The figure shows three views and two pictorial views of one solid part (mm, origin at its lowest corner). Answer the questions. A direction names the side the tool comes from. Give positions to 0.01 mm unless a question says otherwise; leave off trailing zeros. Order: outer loops, then holes, each group sorted by start corner. A loop starts at its lowest first (then second) coordinate and runs counter-clockwise, first axis right, second up. Notation, with made-up numbers: (64.25, 63) - (115.25, 63) arc R28 ccw to (115.25, 84) - close; hole circle Ø11 at (-30.5, 16). An arc over 180 degrees is marked (long way). Answer as CSV lines item,"result". Start each with the question number.
1. Section A-A on z = 28.5 is taken. Give the vertices of the cut face in (x, y).
2. Section B-B on x = 6.5 is taken. Count the separate pieces of the cut face and the enclosed holes in it, and give its area (4 significant figures).
3. Section D-D on z = 6.9 is taken. Give the vertices of the cut face in (x, y).
4. Flat-ended cylindrical pins translate along their axes: pin 1 (2 mm diameter, centred on x = 6.5, z = 24, fed in from +Y); pin 2 (14.5 mm diameter, centred on y = 12.95, z = 6.9, fed in from +X); pin 3 (14.5 mm diameter, centred on x = 29.5, y = 13, fed in from -Z). Find the tip coordinate at first contact, or state that the pin passes through.
5. Which of the six approach directions +Z, -Z, +X, -X, +Y, -Y give full straight-line access (tool end or side, diameter ignored) to the marked faces 5, 6 and 7?
6. Section C-C on y = 22 is taken. Give the vertices of the cut face in (x, z).
7. Consider line 1 along Z through (x, y) = (6.5, 29); line 2 along X through (y, z) = (2.25, 28.5); line 3 along Y through (x, z) = (6.5, 23.25). Determine where each line is inside the solid, lowest interval first. Write a range as [from, to].
8. Determine the mould class of the marked faces 1, 2, 3 and 4 for opening direction Z: +Z half, -Z half, draft (parallel to the pull), parting line (faces both ways), or undercut.
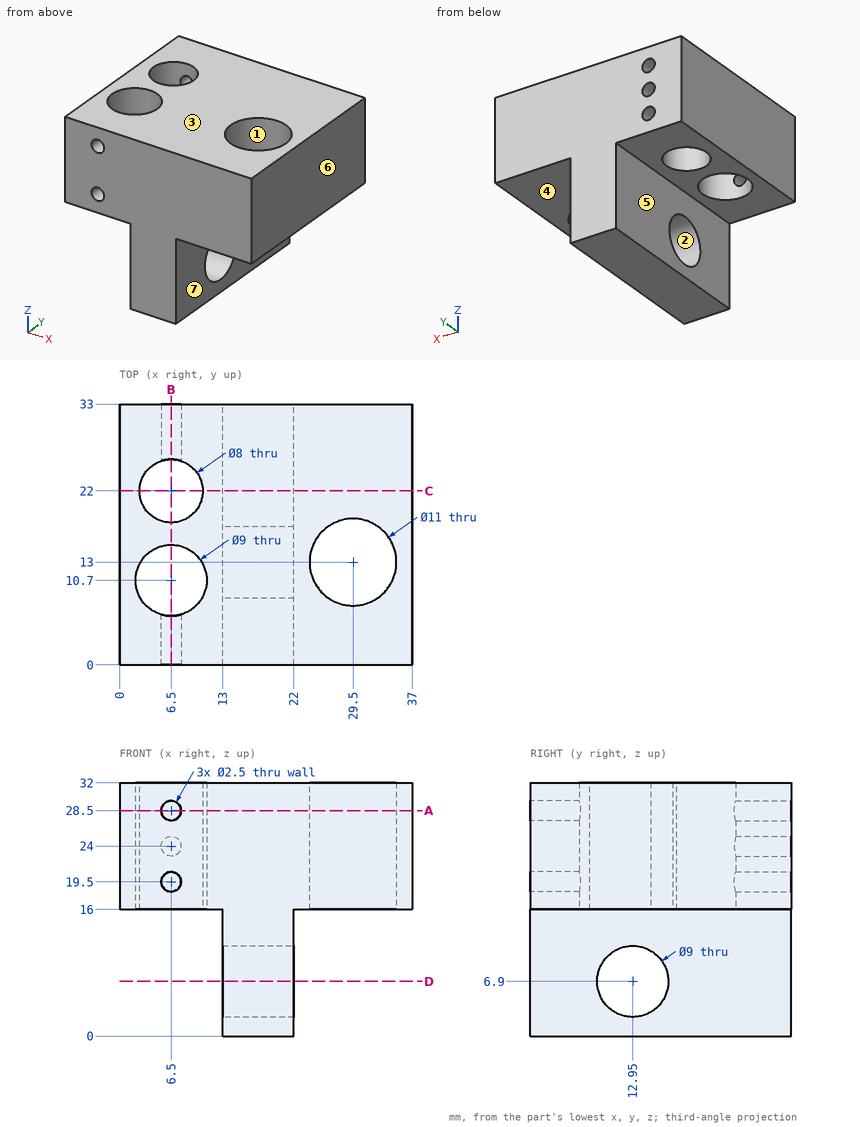
Checks:
1,outline,"(0, 0) - (5.25, 0) - (5.25, 6.38) arc R4.5 cw (long way) to (7.75, 6.38) - (7.75, 0) - (37, 0) - (37, 33) - (7.75, 33) - (7.75, 25.8) arc R4 cw (long way) to (5.25, 25.8) - (5.25, 33) - (0, 33) - close; hole circle Ø11 at (29.5, 13)"
2,separate pieces,"8"
2,enclosed holes,"0"
2,area,"172.5 mm²"
3,outline,"(13, 0) - (22, 0) - (22, 8.45) - (13, 8.45) - close; (13, 17.45) - (22, 17.45) - (22, 33) - (13, 33) - close"
4,pin 1,"stops at y = 18.13"
4,pin 2,"stops at x = 22"
4,pin 3,"stops at z = 16"
5,face 5,"-Z, -X, +Y, -Y"
5,face 6,"+Z, -Z, +X, +Y, -Y"
5,face 7,"-Z, +X, +Y, -Y"
6,outline,"(0, 16) - (2.5, 16) - (2.5, 32) - (0, 32) - close; (10.5, 16) - (13, 16) - (13, 0) - (22, 0) - (22, 16) - (37, 16) - (37, 32) - (10.5, 32) - close"
7,line 1,"z = [16, 18.25], [20.75, 22.75], [25.25, 27.25], [29.75, 32]"
7,line 2,"x = [0, 5.25], [7.75, 37]"
7,line 3,"y = [0, 6.2], [15.2, 18]"
8,face 1,"draft"
8,face 2,"undercut"
8,face 3,"+Z half"
8,face 4,"-Z half"
